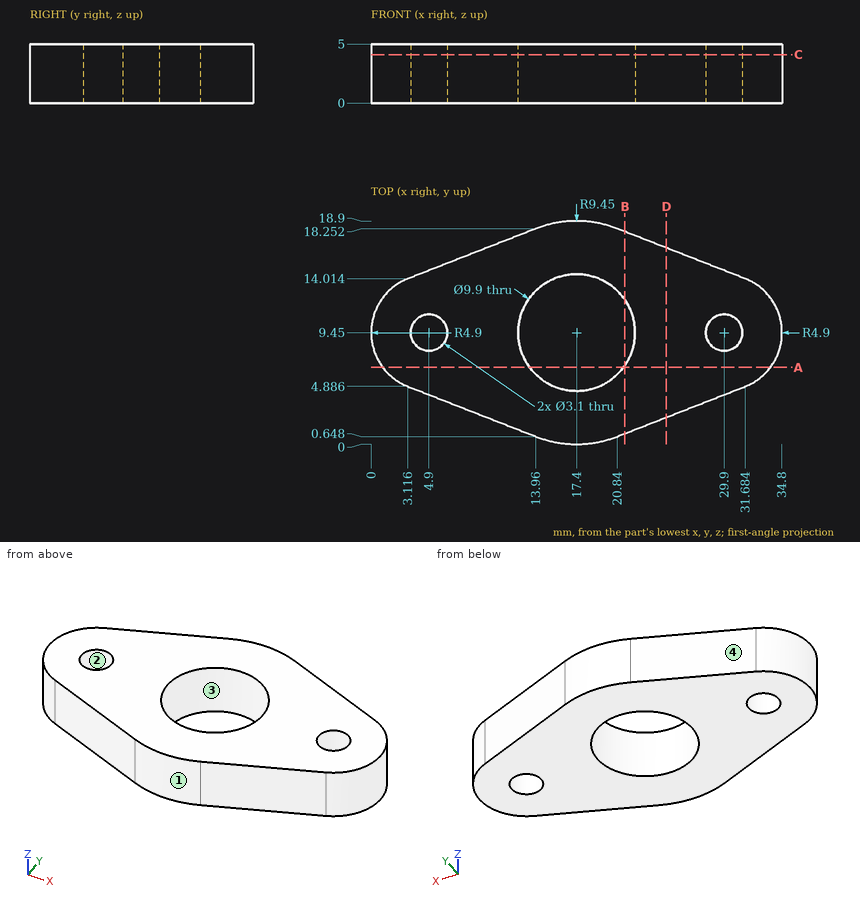
The drawing under review shows one solid part. Ordinate dimensions are in mm from its lowest x, y, z. Give positions to 0.01 mm unless a question says otherwise; leave off trailing zeros. Loops run counter-clockwise (first coordinate to the right, second up) from the corner with the lowest first, then second, coordinate; pieces in that order, holes last. Notation, with made-up numbers: M 14,69.25 L 38,69.25 A29 ccw 38,99.25 Z; hole C 5,25.25 d4. An arc over 180 degrees is marked long. One line per item, written item: value. Start each with the question number.
Q1. For L1, parallel to X at y = 9.5, z = 3.1; L2, parallel to Y at x = 18, z = 2.1; L3, parallel to Y at x = 31, z = 2.2, list the stretches that pass through material, from the lowest coordinate up.
Q2. Add section C-C (z = 4.1). Give the boundary of the cut face in (x, y).
Q3. Clearance check with flat-ended pins moving along their axes: pin 1 Ø1.5 at (x, z) = (23, 3) entering from -Y; pin 2 Ø1.9 at (x, y) = (4.9, 9.45) entering from -Z; pin 3 Ø1.5 at (y, z) = (11, 4) entering from -X. State where each tip first meets the part, or that it passes through.
Q4. Add section D-D (x = 25). Give the boundary of the cut face in (y, z) (1 decimal).
Q5. Add section B-B (x = 21.5). Give the boundary of the cut face in (y, z).
Q6. Add section A-A (y = 6.5). Give the boundary of the cut face in (x, z) (1 decimal), and give its area (3 significant figures).
Q7. Draft analysis for pull direction Y (two halves, no side actions). For the marked faces 1, 2, 3 and 4, state which applies: released by +Y, released by -Y, zero draft, split by the parting line, or undercut.
Reply:
1. L1: 0 to 3.35, 6.45 to 12.45, 22.35 to 28.35, 31.45 to 34.8
1. L2: 0.02 to 4.54, 14.36 to 18.88
1. L3: 4.62 to 8.36, 10.54 to 14.28
2. outline: M 3.12,4.89 L 13.96,0.65 A9.45 ccw 20.84,0.65 L 31.68,4.89 A4.9 ccw 31.68,14.01 L 20.84,18.25 A9.45 ccw 13.96,18.25 L 3.12,14.01 A4.9 ccw Z; hole C 4.9,9.45 d3.1; hole C 17.4,9.45 d9.9; hole C 29.9,9.45 d3.1
3. pin 1: y = 1.2
3. pin 2: through
3. pin 3: x = 0.07
4. outline: M 2.3,0 L 16.6,0 L 16.6,5 L 2.3,5 Z
5. outline: M 0.91,0 L 6.68,0 L 6.68,5 L 0.91,5 Z; M 12.22,0 L 17.99,0 L 17.99,5 L 12.22,5 Z
6. outline: M 1,0 L 13.4,0 L 13.4,5 L 1,5 Z; M 21.4,0 L 33.8,0 L 33.8,5 L 21.4,5 Z
6. area: 124 mm²
7. face 1: released by -Y
7. face 2: undercut
7. face 3: undercut
7. face 4: released by +Y
